The listing builds one solid part. Answer for the finished solid, in the listing's coordinates (mm). Round coordinates to 2 decimals unless told otherwise and drop trailing zeros. Loops run counter-clockwise (first coordinate to the right, second up) from the corner with the lowest first, then second, coordinate; pieces in that order, holes last. Notation, with made-up numbers: (61.5, -27.5) -> (106.5, -27.5) arc R19 cw to (106.5, 0.5) -> close; hole circle Ø3 at (55, 46). An arc over 180 degrees is marked (long way). Use a Markdown table: item, result. Add a question column.
Q1. Section A-A on z = 32 is taken. Give the vertices of the cut face in (x, y).
Q2. Section B-B on y = -1.6 is taken. Give the vertices of the cut face in (x, z), then the cut area to 3 significant figures.
Q3. Given pin 1 Ø3 at (y, z) = (1.5, 35) entering from +X, flat-ended and moving along its own axis, determine where the tip first touches the part or whether it passes through.
Q4. Consider line 1 (Z direction, x = -0.8, y = -2.3); line 2 (Y direction, x = 0.2, z = 184.5). Determine where each line is inside the solid, lowest interval first.
from build123d import *

# Parameters (mm, degrees)
ESBO_O1_W                = 5.7
ESBO_O1_H                = 5.7
RESSALTO_EXTRUS_O1_DEPTH = 19
ESBO_O2_R                = 0.25
RESSALTO_EXTRUS_O2_DEPTH = 220


with BuildPart() as part:
    # Esboço1 → Ressalto-extrusão1 (new body)
    with BuildSketch(Plane.XY):
        Rectangle(ESBO_O1_W, ESBO_O1_H)
    extrude(amount=RESSALTO_EXTRUS_O1_DEPTH)

    # Esboço2 → Ressalto-extrusão2 (add)
    with BuildSketch(Plane.XY.offset(19)):
        with Locations(Location((0, 0, 0), (0, 0, 180))):
            Circle(ESBO_O2_R)
    extrude(amount=RESSALTO_EXTRUS_O2_DEPTH)


solid = part.part
Checked values:
| question | item | result |
|---|---|---|
| 1 | outline | circle Ø0.5 at (0, 0) |
| 2 | outline | (-2.85, 0) -> (2.85, 0) -> (2.85, 19) -> (-2.85, 19) -> close |
| 2 | area | 108 mm2 |
| 3 | pin 1 | stops at x = 0.25 |
| 4 | line 1 | z = 0 to 19 |
| 4 | line 2 | y = -0.15 to 0.15 |
